from build123d import *

# Parameters (mm, degrees)
CROQUIS1_W              = 45.31
CROQUIS1_H              = 20.51
CROQUIS1_R              = 0.8
SALIENTE_EXTRUIR1_DEPTH = 1.58
CROQUIS2_W              = 0.4
CROQUIS2_H              = 0.4
CORTAR_EXTRUIR1_DEPTH   = 50.760954573


with BuildPart() as part:
    # Croquis1 → Saliente-Extruir1 (new body)
    with BuildSketch(Plane(origin=(0, 0, 0), x_dir=(1, 0, 0), z_dir=(0, 1, 0))):
        with Locations((22.655, 10.255)):
            Rectangle(CROQUIS1_W, CROQUIS1_H)
        with Locations(Location((1.4, 19.11, 0), (0, 0, 90))):
            Circle(CROQUIS1_R, mode=Mode.SUBTRACT)
        with Locations(Location((43.91, 19.11, 0), (0, 0, 90))):
            Circle(CROQUIS1_R, mode=Mode.SUBTRACT)
        with Locations(Location((1.4, 1.4, 0), (0, 0, 90))):
            Circle(CROQUIS1_R, mode=Mode.SUBTRACT)
        with Locations(Location((43.91, 1.4, 0), (0, 0, 90))):
            Circle(CROQUIS1_R, mode=Mode.SUBTRACT)
    extrude(amount=SALIENTE_EXTRUIR1_DEPTH)

    # Croquis2 → Cortar-Extruir1 (cut, through all)
    with BuildSketch(Plane.XZ):
        with Locations((21.355, -18.91)):
            Rectangle(CROQUIS2_W, CROQUIS2_H)
        with Locations((18.755, -18.91)):
            Rectangle(CROQUIS2_W, CROQUIS2_H)
        with Locations((23.955, -18.91)):
            Rectangle(CROQUIS2_W, CROQUIS2_H)
        with Locations((26.555, -18.91)):
            Rectangle(CROQUIS2_W, CROQUIS2_H)
    extrude(amount=-CORTAR_EXTRUIR1_DEPTH, mode=Mode.SUBTRACT)


solid = part.part
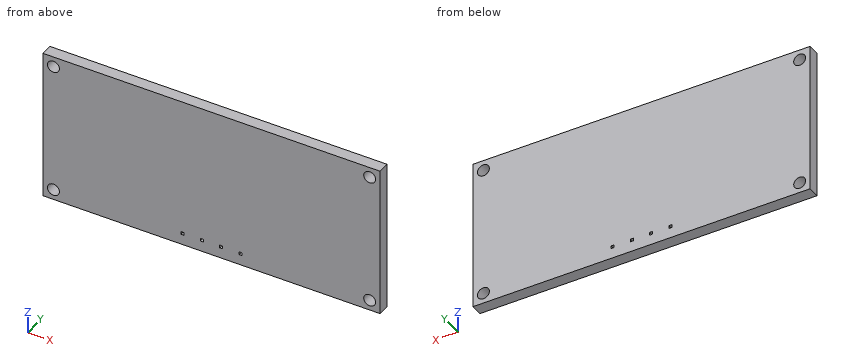
CAD build for the part. Positions are in the model's coordinates, mm. Coordinates: 2 decimals unless noted, no trailing zeros. Loops run counter-clockwise (first coordinate to the right, second up) from the corner with the lowest first, then second, coordinate; pieces in that order, holes last. Notation, with made-up numbers: (13.25, -16) - (23.25, -16) arc R10 ccw to (23.25, -11) - close; hole circle Ø6 at (25, -18.75). An arc over 180 degrees is marked (long way). Use one line per item in the form item = value. Start each with the question number.
1) Flat gauge pin, fed straight in: pin 1 (2.5 mm diameter, centred on x = 43.91, z = -1.4, fed in from -Y). Where does the tip first touch, or does it go through?
2) Drill centre lines: L1, parallel to Z at x = 43.91, y = 0.45; L2, parallel to X at y = 0.8, z = -1.5; L3, parallel to X at y = 0.4, z = -1.75. Where is each one in solid material? Low to high. Write a range as from..to.
3) Band-saw the part on A-A (x = 43.91). Give the cut face in (y, z).
Check values:
q1.pin_1 = 0
q2.L1 = -20.51..-19.91, -18.31..-2.2, -0.6..0
q2.L2 = 0..0.61, 2.19..43.12, 44.7..45.31
q2.L3 = 0..0.68, 2.12..43.19, 44.63..45.31
q3.outline = (0, -20.51) - (1.58, -20.51) - (1.58, -19.91) - (0, -19.91) - close; (0, -18.31) - (1.58, -18.31) - (1.58, -2.2) - (0, -2.2) - close; (0, -0.6) - (1.58, -0.6) - (1.58, 0) - (0, 0) - close
